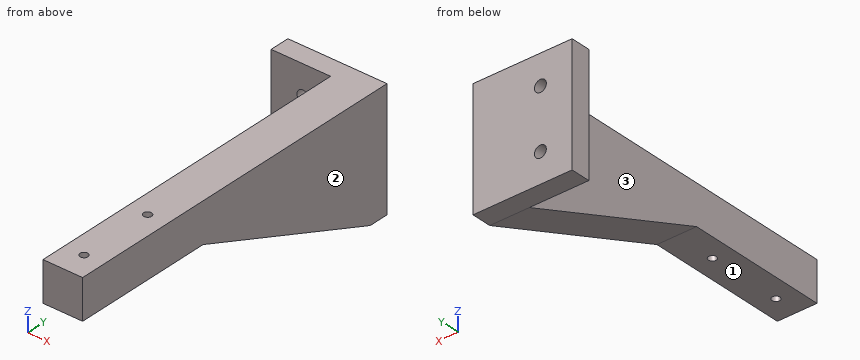
Solid Edge part; units mm, degrees
sketch "Sketch1" plane through (0, 0, 0) normal (0, -1, 0) x (1, 0, 0)
  line L0 (-20, -15) -> (20, -15)
  line L1 (20, -15) -> (20, 15)
  line L2 (20, 15) -> (-20, 15)
  line L3 (-20, 15) -> (-20, -15)
  dimension "D1" = 20
  dimension "D2" = 20
extrude "Protrusion1" add sketch "Sketch1" against normal blind 5
sketch "Sketch2" plane through (0, 0, 0) normal (0, -1, 0) x (1, 0, 0)
  line L0 (-5, -15) -> (5, -15)
  line L1 (5, -15) -> (5, 15)
  line L2 (5, 15) -> (-5, 15)
  line L3 (-5, 15) -> (-5, -15)
extrude "Extrusionsausprägung_2" add sketch "Sketch2" along normal blind 86
sketch "Sketch3" plane through (5, -37.5, 0) normal (1, 0, 0) x (0, 1, 0)
  line L0 (-52.5, 5) -> (-52.5, -15)
  line L1 (-12.5, 5) -> (-52.5, 5)
  line L2 (-12.5, 5) -> (37.5, -15)
  line L3 (37.5, -15) -> (-48.5, -15)
  dimension "D1" = 52.5
  dimension "D2" = 12.5
extrude "Cutout1" cut sketch "Sketch3" against normal through all material side at (5, -89.95, -5)
sketch "Sketch4" plane through (0, -55, 5) normal (0, 0, -1) x (0, 1, 0)
  circle A0 centre (-5.65, 0) radius 1
  circle A1 centre (-24.65, 0) radius 1
  dimension "D1" = 24.65
extrude "Cutout2" cut sketch "Sketch4" against normal through all
sketch "Sketch5" plane through (-12.5, 0, 0) normal (0, -1, 0) x (1, 0, 0)
  circle A0 centre (0.5, 7.5) radius 1.5
  circle A1 centre (0.5, -7.5) radius 1.5
  dimension "D1" = 0.5
  dimension "D2" = 0.5
extrude "Cutout3" cut sketch "Sketch5" against normal through all
sketch "Sketch6" plane through (12.5, 0, 0) normal (0, -1, 0) x (1, 0, 0)
  line L0 (7.5, 15) -> (-7.5, 15)
  line L1 (-7.5, 15) -> (-7.5, -15)
  line L2 (-7.5, -15) -> (7.5, -15)
  line L3 (7.5, -15) -> (7.5, 15)
extrude "Cutout4" cut sketch "Sketch6" against normal through all
properties material "Nylon, allgemein"
Could you check a few things on this model? Use its own coordinates, in mm. Face numbers are marked on the shaded views. A direction names the side the tool comes from. Coordinates: 2 decimals unless noted, no trailing zeros. Loops run counter-clockwise (first coordinate to the right, second up) from the corner with the lowest first, then second, coordinate; pieces in that order, holes last.
1. Imagine slicing it at D-D (z = 7.5). Please give me the cut outline in (x, y).
2. Imagine slicing it at C-C (y = -60.65). Please give me the cut outline in (x, z), and give its area (3 significant figures).
3. For P1, Ø8, axis at y = -5, z = 4.5, coming from the -X side; P2, Ø11, axis at x = -1.5, y = -72.5, coming from the -Z side; P3, Ø3.5, axis at x = -12, z = -7.5, coming from the -Y side, each with a flat end and sliding along its axis, tell me the tip position at first contact or that it passes through.
4. For the marked faces 1, 2 and 3, which set-ups out of +Z, -Z, +X, -X, +Y, -Y let a thin tool reach every point of the face, with its end or its side?
5. I need wall thicknesses on L1, parallel to Z at x = -12, y = 1.15; L2, parallel to Y at x = -8, z = -13.5; L3, parallel to X at y = -36, z = 13.5. Which ranges of each line are inside material? Lowest first, please.
6. Imagine slicing it at B-B (x = -12). Please give me the cut outline in (y, z).
7. Imagine slicing it at A-A (z = -7.5). Please give me the cut outline in (x, y), and give its area (4 significant figures).
Computed values:
1. outline: (-20, 0) - (-13.5, 0) - (-13.5, 5) - (-20, 5) - close; (-10.5, 0) - (-5, 0) - (-5, -86) - (5, -86) - (5, 5) - (-10.5, 5) - close; hole circle Ø2 at (0, -79.65); hole circle Ø2 at (0, -60.65)
2. outline: (-5, 5) - (-1, 5) - (-1, 15) - (-5, 15) - close; (1, 5) - (5, 5) - (5, 15) - (1, 15) - close
2. area: 80.0 mm2
3. P1: stops at x = -5
3. P2: stops at z = 5
3. P3: stops at y = 0
4. face 1: -Z, +X, -X, -Y
4. face 2: +Z, -Z, +X, +Y, -Y
4. face 3: +Z, -Z, -X, -Y
5. L1: z = -15 to -9, -6 to 6, 9 to 15
5. L2: y = 0 to 5
5. L3: x = -5 to 5
6. outline: (0, -15) - (5, -15) - (5, -9) - (0, -9) - close; (0, -6) - (5, -6) - (5, 6) - (0, 6) - close; (0, 9) - (5, 9) - (5, 15) - (0, 15) - close
7. outline: (-20, 0) - (-13.5, 0) - (-13.5, 5) - (-20, 5) - close; (-10.5, 0) - (-5, 0) - (-5, -18.75) - (5, -18.75) - (5, 5) - (-10.5, 5) - close
7. area: 297.5 mm2
